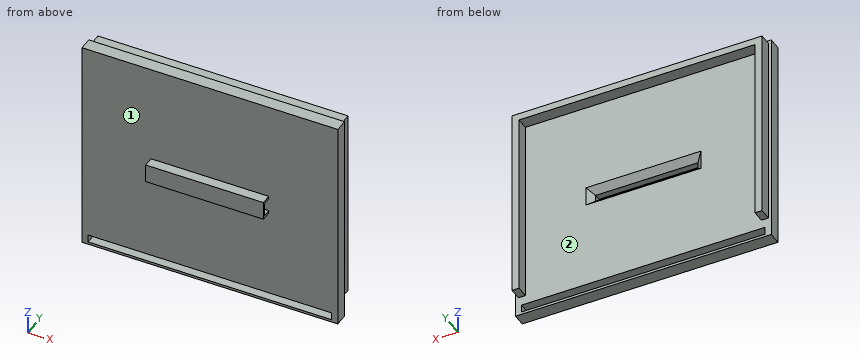
from build123d import *

# Parameters (mm, degrees)
CROQUIS1_W              = 200
CROQUIS1_H              = 170
SALIENTE_EXTRUIR1_DEPTH = 10
SALIENTE_EXTRUIR2_DEPTH = 19.5
CROQUIS2_W              = 169.5
CROQUIS2_H              = 6
CROQUIS2_W_2            = 5.25
CORTAR_EXTRUIR1_DEPTH   = 20
CROQUIS3_W              = 80
CROQUIS3_H              = 5
CORTAR_EXTRUIR2_DEPTH   = 10
CHAFL_N1_SIZE           = 5
CROQUIS4_W              = 92
CROQUIS4_H              = 14.5
CROQUIS4_W_2            = 86
CROQUIS4_H_2            = 8.5
SALIENTE_EXTRUIR3_DEPTH = 6
CROQUIS5_W              = 92
CROQUIS5_H              = 14.5
SALIENTE_EXTRUIR4_DEPTH = 2
CORTAR_EXTRUIR3_DEPTH   = 90


with BuildPart() as part:
    # Croquis1 → Saliente-Extruir1 (new body)
    with BuildSketch(Plane(origin=(0, 0, 0), x_dir=(1, 0, 0), z_dir=(0, 1, 0))):
        Rectangle(CROQUIS1_W, CROQUIS1_H)
    extrude(amount=SALIENTE_EXTRUIR1_DEPTH)

    # Croquis1<4> → Saliente-Extruir2 (add)
    with BuildSketch(Plane(origin=(0, 0, 0), x_dir=(1, 0, 0), z_dir=(0, 1, 0))):
        Polygon((97.75, 69.75), (97.75, -82.75), (-97.75, -82.75), (-97.75, 69.75), (-92.25, 69.75), (-92.25, -77.25), (92.25, -77.25), (92.25, 69.75), align=None)
    extrude(amount=SALIENTE_EXTRUIR2_DEPTH)

    # Croquis2 → Cortar-Extruir1 (cut)
    with BuildSketch(Plane(origin=(0, 10, 0), x_dir=(1, 0, 0), z_dir=(0, 1, 0))):
        with Locations((0, 80)):
            Rectangle(CROQUIS2_W, CROQUIS2_H)
        with Locations((-87.375, 80)):
            Rectangle(CROQUIS2_W_2, CROQUIS2_H)
        with Locations((-92.625, 80)):
            Rectangle(CROQUIS2_W_2, CROQUIS2_H)
        with Locations((87.375, 80)):
            Rectangle(CROQUIS2_W_2, CROQUIS2_H)
        with Locations((92.625, 80)):
            Rectangle(CROQUIS2_W_2, CROQUIS2_H)
    extrude(amount=-CORTAR_EXTRUIR1_DEPTH, mode=Mode.SUBTRACT)

    # Croquis3 → Cortar-Extruir2 (cut)
    with BuildSketch(Plane.XZ):
        Rectangle(CROQUIS3_W, CROQUIS3_H)
    extrude(amount=-CORTAR_EXTRUIR2_DEPTH, mode=Mode.SUBTRACT)

    # Chaflán1
    chafl_n1_edges = [part.edges().sort_by_distance(p)[0] for p in [
        (0, 10, -2.5),
        (-40, 10, 0),
        (0, 10, 2.5),
        (40, 10, 0),
    ]]
    chamfer(chafl_n1_edges, length=CHAFL_N1_SIZE)

    # Croquis4 → Saliente-Extruir3 (add)
    with BuildSketch(Plane.XZ):
        Rectangle(CROQUIS4_W, CROQUIS4_H)
        Rectangle(CROQUIS4_W_2, CROQUIS4_H_2, mode=Mode.SUBTRACT)
    extrude(amount=SALIENTE_EXTRUIR3_DEPTH)

    # Croquis5 → Saliente-Extruir4 (add)
    with BuildSketch(Plane.XZ.offset(6)):
        Rectangle(CROQUIS5_W, CROQUIS5_H)
    extrude(amount=SALIENTE_EXTRUIR4_DEPTH)

    # Croquis6 → Cortar-Extruir3 (cut)
    with BuildSketch(Plane(origin=(46, 0, 0), x_dir=(0, 0, -1), z_dir=(1, 0, 0))):
        Polygon((5.25, 0), (5.25, -6), (-5.25, -6), (-5.25, 0), (0, 0), align=None)
    extrude(amount=-CORTAR_EXTRUIR3_DEPTH, mode=Mode.SUBTRACT)


solid = part.part
Work out the finished part from the listing and answer in its coordinate system (mm). Face numbers are marked on the shaded views. Round coordinates to 2 decimals unless told otherwise and drop trailing zeros. Write each loop counter-clockwise with the first axis right and the second up, starting at its lowest first coordinate (ties: lowest second). Pieces come first, ordered by that corner, then holes. Notation, with made-up numbers: M 61,57.25 L 107,57.25 A22 ccw 107,90.25 Z; hole C 69,-1 d9. An arc over 180 degrees is marked long. Use a Markdown table: item, result.
1) Determine the mould class of the marked faces 1 and 2 for opening direction X: pulls with the +X half, pulls with the -X half, needs draft (parallel to the pull), parting line crosses it, or undercut.
Taken from the geometry:
| item | result |
|---|---|
| face 1 | needs draft |
| face 2 | undercut |
2) The part is cut by section D-D on x = 4. Give the vertices of the cut face in (y, z), plus the area to 3 significant figures.
Taken from the geometry:
| item | result |
|---|---|
| outline | M -8,-7.25 L 0,-7.25 L 0,-77 L 10,-77 L 10,-7.5 L 5,-2.5 L 0,-2.5 L 0,-5.25 L -6,-5.25 L -6,5.25 L 0,5.25 L 0,2.5 L 5,2.5 L 10,7.5 L 10,77.25 L 19.5,77.25 L 19.5,82.75 L 10,82.75 L 10,85 L 0,85 L 0,7.25 L -8,7.25 Z; M 0,-85 L 10,-85 L 10,-83 L 0,-83 Z |
| area | 1,670 mm2 |
3) The part is cut by section A-A on x = -80.5. Give the vertices of the cut face in (y, z), plus the area to 3 significant figures.
Taken from the geometry:
| item | result |
|---|---|
| outline | M 0,-85 L 10,-85 L 10,-83 L 0,-83 Z; M 0,-77 L 10,-77 L 10,77.25 L 19.5,77.25 L 19.5,82.75 L 10,82.75 L 10,85 L 0,85 Z |
| area | 1,690 mm2 |
4) The part is cut by section C-C on z = 66.5. Give the vertices of the cut face in (x, y), plus the area to 3 significant figures.
Taken from the geometry:
| item | result |
|---|---|
| outline | M -100,0 L 100,0 L 100,10 L 97.75,10 L 97.75,19.5 L 92.25,19.5 L 92.25,10 L -92.25,10 L -92.25,19.5 L -97.75,19.5 L -97.75,10 L -100,10 Z |
| area | 2,100 mm2 |
5) The part is cut by section B-B on y = 15. Give the vertices of the cut face in (x, z).
Taken from the geometry:
| item | result |
|---|---|
| outline | M -97.75,-69.75 L -92.25,-69.75 L -92.25,77.25 L 92.25,77.25 L 92.25,-69.75 L 97.75,-69.75 L 97.75,82.75 L -97.75,82.75 Z |
6) Flat-ended cylindrical pins translate along their axes: pin 1 (10 mm diameter, centred on x = -29, z = -13.5, fed in from -Y); pin 2 (1.5 mm diameter, centred on x = -51, z = 12, fed in from +Y); pin 3 (8 mm diameter, centred on y = 12.5, z = -42, fed in from -X); pin 4 (5 mm diameter, centred on x = -38.5, y = 13, fed in from -Z). Find the tip coordinate at first contact, or state that the pin passes through.
Taken from the geometry:
| item | result |
|---|---|
| pin 1 | stops at y = 0 |
| pin 2 | stops at y = 10 |
| pin 3 | stops at x = -100 |
| pin 4 | stops at z = 77.25 |
7) Consider line 1 (Z direction, x = -17.5, y = -3.5); line 2 (X direction, y = 16.5, z = -60); line 3 (Z direction, x = -18, y = 5.75). Determine where each line is inside the solid, lowest interval first. Write a range as [from, to].
Taken from the geometry:
| item | result |
|---|---|
| line 1 | z = [-7.25, -5.25], [5.25, 7.25] |
| line 2 | x = [-97.75, -92.25], [92.25, 97.75] |
| line 3 | z = [-85, -83], [-77, -3.25], [3.25, 85] |
